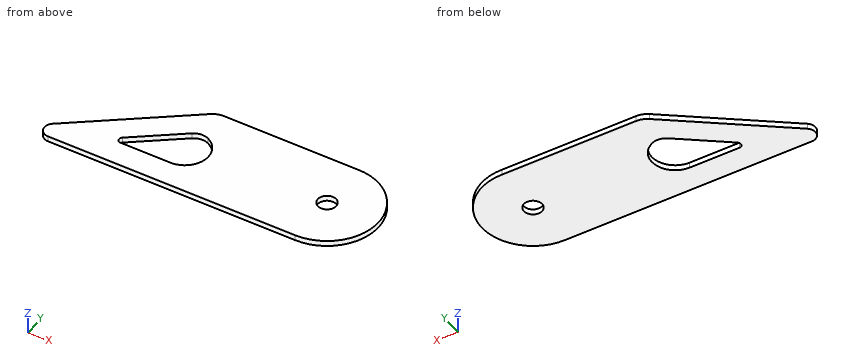
```python
from build123d import *

# Parameters (mm, degrees)
SKETCH2_R           = 25
BOSS_EXTRUDE1_DEPTH = 7.5


with BuildPart() as part:
    # Sketch2 → Boss-Extrude1 (new body, symmetric)
    with BuildSketch(Plane.XY):
        with BuildLine():
            Line((-398.468541926, -10.340558916), (-691.280931438, -235.14913744))
            ThreePointArc((-691.280931438, -235.14913744), (-699.728704435, -263.018042843), (-676.056537091, -279.978857982))
            Line((-676.056537091, -279.978857982), (2.432964843, -279.978857982))
            ThreePointArc((2.432964843, -279.978857982), (142.427679239, -138.762329632), (0, 0))
            Line((0, 0), (-368.019753232, 0))
            ThreePointArc((-368.019753232, 0), (-384.098122954, -2.655665311), (-398.468541926, -10.340558916))
        make_face()
        with Locations((2.432964843, -139.978857982)):
            Circle(SKETCH2_R, mode=Mode.SUBTRACT)
        with BuildLine():
            Line((-526.980915272, -192.046969766), (-398.014187587, -93.031942512))
            ThreePointArc((-398.014187587, -93.031942512), (-377.665337115, -84.961022387), (-356.115398822, -88.810129655))
            ThreePointArc((-356.115398822, -88.810129655), (-321.919160325, -160.522945456), (-384.098122954, -209.978857982))
            Line((-384.098122954, -209.978857982), (-520.891157533, -209.978857982))
            ThreePointArc((-520.891157533, -209.978857982), (-530.360024471, -203.194531927), (-526.980915272, -192.046969766))
        make_face(mode=Mode.SUBTRACT)
    extrude(amount=BOSS_EXTRUDE1_DEPTH, both=True)


solid = part.part
```
The model under review builds one solid part; all positions refer to its coordinate system, in mm. Round coordinates to 2 decimals unless told otherwise and drop trailing zeros. Loops run counter-clockwise (first coordinate to the right, second up) from the corner with the lowest first, then second, coordinate; pieces in that order, holes last. Notation, with made-up numbers: M 89.5,22.5 L 148.5,22.5 A17 ccw 148.5,48.5 Z; hole C 3.25,4 d9. An arc over 180 degrees is marked long. Answer as a JSON object with one key per item and string values.
(1) Clearance check with flat-ended pins moving along their axes: P1, Ø2, axis at x = -44.5, z = -3, coming from the +Y side; P2, Ø4, axis at y = -83.5, z = 5.5, coming from the +X side; P3, Ø1.5, axis at x = -535, z = -0.5, coming from the +Y side. State where each tip first meets the part, or that it passes through.
Resolved:
{"P1": "y = 0", "P2": "x = 131.4", "P3": "y = -114.59"}
(2) To check wall thickness, follow line 1 along X through (y, z) = (-124, -6.5); line 2 along X through (y, z) = (-156.5, 1.5); line 3 along Y through (x, z) = (-395.5, -4.75). State the ranges of each line that lie inside material, in increasing order.
Resolved:
{"line 1": "-546.51 to -438.35, -324.25 to -16.79, 21.66 to 141.52", "line 2": "-588.84 to -480.68, -321.13 to -16.33, 21.2 to 141.45", "line 3": "-279.98 to -209.98, -91.25 to -8.23"}
(3) Take a section at D-D on y = -260.5. Give the boundary of the cut face in (x, z), and give its area (3 significant figures).
Resolved:
{"outline": "M -700.44,-7.5 L 73.67,-7.5 L 73.67,7.5 L -700.44,7.5 Z", "area": "11,600 mm²"}
(4) Take a section at A-A on x = -413. Give the boundary of the cut face in (y, z).
Resolved:
{"outline": "M -279.98,-7.5 L -209.98,-7.5 L -209.98,7.5 L -279.98,7.5 Z; M -104.54,-7.5 L -21.5,-7.5 L -21.5,7.5 L -104.54,7.5 Z"}
(5) Take a section at B-B on y = -150. Give the boundary of the cut face in (x, z).
Resolved:
{"outline": "M -580.37,-7.5 L -472.21,-7.5 L -472.21,7.5 L -580.37,7.5 Z; M -320.4,-7.5 L -20.47,-7.5 L -20.47,7.5 L -320.4,7.5 Z; M 25.34,-7.5 L 142.07,-7.5 L 142.07,7.5 L 25.34,7.5 Z"}
(6) Take a section at C-C on z = -4. Give the boundary of the cut face in (x, y), and give its area (3 significant figures).
Resolved:
{"outline": "M -691.28,-235.15 A25 ccw -676.06,-279.98 L 2.43,-279.98 A140 ccw long 0,0 L -368.02,0 A50 ccw -398.47,-10.34 Z; hole M -526.98,-192.05 A10 ccw -520.89,-209.98 L -384.1,-209.98 A63.82 ccw -356.12,-88.81 A40 ccw -398.01,-93.03 Z; hole C 2.43,-139.98 d50", "area": "170,000 mm²"}
